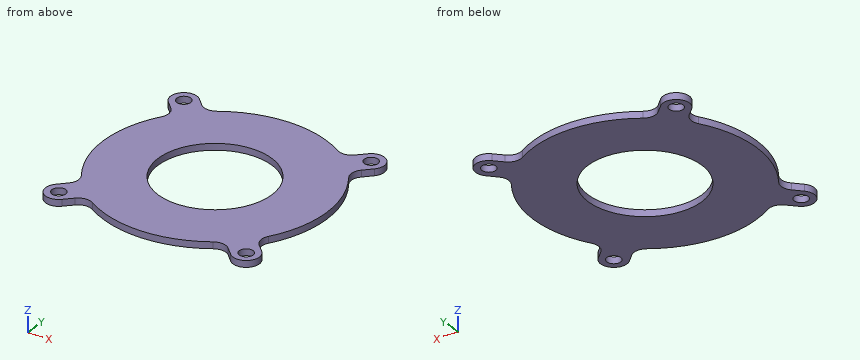
```python
from build123d import *

# Parameters (mm, degrees)
SKETCH_1_R      = 2.1
SKETCH_1_R_2    = 17.225
EXTRUDE_1_DEPTH = 2


with BuildPart() as part:
    # 草图1 → 凸台-拉伸1 (new body)
    with BuildSketch(Plane.XY):
        with BuildLine():
            Line((49.221320344, -54.878174593), (46.870064467, -52.526918716))
            ThreePointArc((46.870064467, -52.526918716), (44.466937039, -51.378020085), (41.875216055, -51.992814233))
            ThreePointArc((41.875216055, -51.992814233), (23.55, -57.385), (5.224783944, -51.992814233))
            ThreePointArc((5.224783944, -51.992814233), (2.633062961, -51.378020085), (0.229935533, -52.526918716))
            Line((0.229935533, -52.526918716), (-2.121320344, -54.878174593))
            ThreePointArc((-2.121320344, -54.878174593), (-7.778174593, -54.878174593), (-7.778174593, -49.221320343))
            Line((-7.778174593, -49.221320343), (-5.426918716, -46.870064466))
            ThreePointArc((-5.426918716, -46.870064466), (-4.278020085, -44.466937039), (-4.892814233, -41.875216055))
            ThreePointArc((-4.892814233, -41.875216055), (-10.285, -23.55), (-4.892814233, -5.224783944))
            ThreePointArc((-4.892814233, -5.224783944), (-4.278020085, -2.633062961), (-5.426918716, -0.229935533))
            Line((-5.426918716, -0.229935533), (-7.778174593, 2.121320344))
            ThreePointArc((-7.778174593, 2.121320344), (-7.778174593, 7.778174593), (-2.121320343, 7.778174593))
            Line((-2.121320343, 7.778174593), (0.229935534, 5.426918716))
            ThreePointArc((0.229935534, 5.426918716), (2.633062962, 4.278020085), (5.224783945, 4.892814234))
            ThreePointArc((5.224783945, 4.892814234), (23.55, 10.285), (41.875216056, 4.892814233))
            ThreePointArc((41.875216056, 4.892814233), (44.466937039, 4.278020085), (46.870064467, 5.426918716))
            Line((46.870064467, 5.426918716), (49.221320344, 7.778174593))
            ThreePointArc((49.221320344, 7.778174593), (54.878174593, 7.778174593), (54.878174593, 2.121320344))
            Line((54.878174593, 2.121320344), (52.526918716, -0.229935533))
            ThreePointArc((52.526918716, -0.229935533), (51.378020085, -2.633062961), (51.992814234, -5.224783945))
            ThreePointArc((51.992814234, -5.224783945), (57.385, -23.55), (51.992814233, -41.875216055))
            ThreePointArc((51.992814233, -41.875216055), (51.378020085, -44.466937039), (52.526918716, -46.870064467))
            Line((52.526918716, -46.870064467), (54.878174593, -49.221320344))
            ThreePointArc((54.878174593, -49.221320344), (54.878174593, -54.878174593), (49.221320344, -54.878174593))
        make_face()
        with Locations((52.049747468, -52.049747468)):
            Circle(SKETCH_1_R, mode=Mode.SUBTRACT)
        with Locations((-4.949747468, -52.049747468)):
            Circle(SKETCH_1_R, mode=Mode.SUBTRACT)
        with Locations((-4.949747468, 4.949747468)):
            Circle(SKETCH_1_R, mode=Mode.SUBTRACT)
        with Locations((52.049747468, 4.949747468)):
            Circle(SKETCH_1_R, mode=Mode.SUBTRACT)
        with Locations((23.55, -23.55)):
            Circle(SKETCH_1_R_2, mode=Mode.SUBTRACT)
    extrude(amount=EXTRUDE_1_DEPTH)


solid = part.part
```
Work out the finished part from the listing and answer in its coordinate system (mm). Coordinates: 2 decimals unless noted, no trailing zeros. Order: outer loops, then holes, each group sorted by start corner. A loop starts at its lowest first (then second) coordinate and runs counter-clockwise, first axis right, second up. Notation, with made-up numbers: M 61,63 L 73,63 A21 cw 73,70 Z; hole C 5,50 d5. An arc over 180 degrees is marked long. Use CSV: the item, a comma, the result in double quotes.
1) Section A-A on y = -23.55 is taken. Write down the section's boundary in (x, z) (3 decimals).
Worked out:
outline,"M -10.285,0 L 6.325,0 L 6.325,2 L -10.285,2 Z; M 40.775,0 L 57.385,0 L 57.385,2 L 40.775,2 Z"
2) A flat-ended cylindrical pin translates along its axis: pin 1 Ø1 at (x, z) = (7.5, 1.5) entering from +Y. Find the tip coordinate at first contact, or state that the pin passes through.
Worked out:
pin 1,"stops at y = 6.5"
3) Section B-B on x = 23.55 is taken. Write down the section's boundary in (y, z) (3 decimals), plus the area to 3 significant figures.
Worked out:
outline,"M -57.385,0 L -40.775,0 L -40.775,2 L -57.385,2 Z; M -6.325,0 L 10.285,0 L 10.285,2 L -6.325,2 Z"
area,"66.4 mm^2"
4) Section C-C on z = 1.55 is taken. Count the separate pieces of the cut face and the enclosed holes in it, plus the area to 3 significant figures.
Worked out:
separate pieces,"1"
enclosed holes,"5"
area,"2,940 mm^2"
5) Consider line 1 (Y direction, x = -5, z = 0.9); line 2 (X direction, y = 6.5, z = 0.7); line 3 (Y direction, x = -5.5, z = 1.75). Determine where each line is inside the solid, lowest interval first. Write a range as [from, to].
Worked out:
line 1,"y = [-56.05, -54.15], [-49.95, -46.37], [-41.71, -5.39], [-0.73, 2.85], [7.05, 8.95]"
line 2,"x = [-8.64, -6.37], [-3.53, -0.84], [8, 39.1], [47.94, 50.63], [53.47, 55.74]"
line 3,"y = [-56.01, -54.08], [-50.02, -46.94], [-40.9, -6.2], [-0.16, 2.92], [6.98, 8.91]"
